Geometry check sheet. Reference: the model listing, model coordinates, mm. A direction names the side the tool comes from. Give positions to 0.01 mm unless a question says otherwise; leave off trailing zeros. Order: outer loops, then holes, each group sorted by start corner. A loop starts at its lowest first (then second) coordinate and runs counter-clockwise, first axis right, second up. Notation, with made-up numbers: M 32,-38.5 L 56,-38.5 A18 cw 56,-30.5 Z; hole C 54,8.5 d11. An arc over 180 degrees is marked long. Answer as a JSON object with one key per item and string values. Group by question number.
from build123d import *

# Parameters (mm, degrees)
SKETCH_W          = 3.32
SKETCH_H          = 32.28
PAD_DEPTH         = 3
PAD001_DEPTH      = 4
SKETCH002_W       = 3.32
SKETCH002_H       = 2
PAD002_DEPTH      = 2.01
FILLET_R          = 1.99
FILLET001_R       = 1.99
SKETCH003_W       = 11.8
SKETCH003_H       = 6.88
PAD003_DEPTH      = 1.5
SKETCH006_W       = 4.25
SKETCH006_H       = 4.4
PAD005_DEPTH      = 1.56
PAD005_DEPTH_BACK = 1.56
SKETCH007_W       = 2.24
SKETCH007_H       = 6.88
PAD006_DEPTH      = 0.92
POCKET_DEPTH      = 5
SKETCH009_R       = 0.72
PAD007_DEPTH      = 5
SKETCH010_R       = 0.72
PAD008_DEPTH      = 5
SKETCH011_R       = 0.8
POCKET001_DEPTH   = 5
SKETCH012_R       = 0.95
POCKET002_DEPTH   = 5


with BuildPart() as part:
    # Sketch → Pad (new body)
    with BuildSketch(Plane.XY):
        Rectangle(SKETCH_W, SKETCH_H)
    extrude(amount=PAD_DEPTH)

    # Sketch001 (on Face5 of Pad) → Pad001 (join)
    with BuildSketch(Plane(origin=(0, 0, 0), x_dir=(1, 0, 0), z_dir=(0, 0, -1))):
        Polygon((1.66, 6.275), (1.66, 11.275), (0, 11.275), (0, 9.385), (-1.66, 9.385), (-1.66, 7.965), (0, 7.965), (0, 6.275), align=None)
    pad001 = extrude(amount=PAD001_DEPTH)

    # Mirrored: Pad001 across Sketch001 H_Axis
    add(pad001.mirror(Plane(origin=(0, 0, 0), x_dir=(0, 0, -1), z_dir=(0, -1, 0))))

    # Sketch002 (on Face6 of Mirrored) → Pad002 (join)
    with BuildSketch(Plane.XZ.offset(16.14)):
        with Locations((0, 0.5)):
            Rectangle(SKETCH002_W, SKETCH002_H)
    pad002 = extrude(amount=PAD002_DEPTH)

    # Fillet
    fillet_edges = [part.edges().sort_by_distance(p)[0] for p in [
        (0, -18.15, 1.5),
    ]]
    fillet(fillet_edges, radius=FILLET_R)

    # Mirrored001: Pad002 across XZ
    add(pad002.mirror(Plane.XZ))

    # Fillet001
    fillet001_edges = [part.edges().sort_by_distance(p)[0] for p in [
        (0, 18.15, 1.5),
    ]]
    fillet(fillet001_edges, radius=FILLET001_R)

    # Sketch003 (on Face23 of Fillet001) → Pad003 (join)
    with BuildSketch(Plane(origin=(0, 0, -0.5), x_dir=(1, 0, 0), z_dir=(0, 0, -1))):
        with Locations((-1.64, 19.58)):
            Rectangle(SKETCH003_W, SKETCH003_H)
    pad003 = extrude(amount=PAD003_DEPTH)

    # Mirrored002: Pad003 across XZ
    add(pad003.mirror(Plane.XZ))

    # Sketch006 → Pad005 (join, two sides)
    with BuildSketch(Plane.XZ) as pad005_sk:
        with Locations((2.125, -0.7)):
            Rectangle(SKETCH006_W, SKETCH006_H)
    extrude(amount=PAD005_DEPTH)
    extrude(pad005_sk.sketch, amount=-PAD005_DEPTH_BACK)

    # Sketch007 (on Face56 of Pad005) → Pad006 (join)
    with BuildSketch(Plane(origin=(0, 0, -2), x_dir=(1, 0, 0), z_dir=(0, 0, -1))):
        with Locations((3.14, 19.58)):
            Rectangle(SKETCH007_W, SKETCH007_H)
    pad006 = extrude(amount=PAD006_DEPTH)

    # Mirrored003: Pad006 across XZ
    add(pad006.mirror(Plane.XZ))

    # Sketch008 (on Face43 of Mirrored003) → Pocket (cut)
    with BuildSketch(Plane.XY.offset(-0.5)):
        Polygon((4.26, -16.14), (4.26, -23.02), (-0.14, -23.02), align=None)
    pocket = extrude(amount=-POCKET_DEPTH, mode=Mode.SUBTRACT)

    # Mirrored004: Pocket across XZ
    add(pocket.mirror(Plane.XZ), mode=Mode.SUBTRACT)

    # Sketch009 (on Face59 of Mirrored004) → Pad007 (join)
    with BuildSketch(Plane(origin=(0, -16.14, 0), x_dir=(-1, 0, 0), z_dir=(0, 1, 0))):
        with Locations((-3.54, -2.2)):
            Circle(SKETCH009_R)
    pad007 = extrude(amount=PAD007_DEPTH)

    # Mirrored005: Pad007 across XZ
    add(pad007.mirror(Plane.XZ))

    # Sketch010 (on Face35 of Mirrored005) → Pad008 (join)
    with BuildSketch(Plane(origin=(0, 1.56, 0), x_dir=(-1, 0, 0), z_dir=(0, 1, 0))):
        with Locations((-3.53, -2.18)):
            Circle(SKETCH010_R)
    pad008 = extrude(amount=PAD008_DEPTH)

    # Mirrored006: Pad008 across XZ
    add(pad008.mirror(Plane.XZ))

    # Sketch011 (on Face2 of Mirrored006) → Pocket001 (cut)
    with BuildSketch(Plane.XY.offset(-0.5)):
        with Locations((-5.74, 20.12)):
            Circle(SKETCH011_R)
    pocket001 = extrude(amount=-POCKET001_DEPTH, mode=Mode.SUBTRACT)

    # Mirrored007: Pocket001 across XZ
    add(pocket001.mirror(Plane.XZ), mode=Mode.SUBTRACT)

    # Sketch012 (on Face2 of Mirrored007) → Pocket002 (cut)
    with BuildSketch(Plane.XY.offset(-0.5)):
        with Locations((-1.81, 20.12)):
            Circle(SKETCH012_R)
    pocket002 = extrude(amount=-POCKET002_DEPTH, mode=Mode.SUBTRACT)

    # Mirrored008: Pocket002 across XZ
    add(pocket002.mirror(Plane.XZ), mode=Mode.SUBTRACT)


solid = part.part
1. Release check for a two-part mould opening along Y. For faces 1 (the flat face through (2.03, -19.63, -1.42)), 2 (the flat face through (0, 0, -1)), 3 (the cylindrical face through (0.023, 17.552, 0.933)), 4 (the flat face through (0, 10, -2)) record: released by +Y, released by -Y, zero draft, split by the parting line, or undercut.
2. Thickness scan on line 1 along Y through (x, z) = (-5.74, -1.3); line 2 along Y through (x, z) = (-1.81, -1.35); line 3 along X through (y, z) = (-11, 1.5). Record the ranges inside material, lowest first. Write a range as [from, to].
3. Cross-section at D-D (y = -20.12). Record the cut outline in (x, z), and give its area (3 significant figures).
4. Cross-section at C-C (x = -2.25). Record the cut outline in (y, z), and give its area (3 significant figures).
5. Cross-section at B-B (y = -13). Record the cut outline in (x, z).
6. Access from +Z, -Z, +X, -X, +Y, -Y to the whole of each face (thin tool, end or side, straight path). Record for faces 5 (the cylindrical face through (2.843, -4.025, -1.964)), 6 (the flat face through (2.03, 19.63, -1.42)), 7 (the flat face through (4, 6.56, -2)), 8 (the flat face through (0, -16.14, 2)), 9 (the flat face through (-1, -7.965, -2)).
7. Cross-section at A-A (x = -4.5). Record the cut outline in (y, z), and give its area (3 significant figures).
8. Depth check by flat-ended pin: pin 1 (0.8 mm diameter, centred on x = 4, z = -2.5, fed in from -Y); pin 2 (3.5 mm diameter, centred on x = 2.5, y = -0.5, fed in from -Z); pin 3 (5 mm diameter, centred on x = -2.5, y = 12, fed in from +Z); pin 4 (2 mm diameter, centred on x = 3, z = -1.5, fed in from -Y). Enter the tip coordinate at first touch or a pass-through.
Report:
{
 "1": {"face 1": "released by -Y", "face 2": "undercut", "face 3": "released by +Y", "face 4": "undercut"},
 "2": {"line 1": "y = [-23.02, -20.92], [-19.32, -16.14], [16.14, 19.32], [20.92, 23.02]", "line 2": "y = [-23.02, -21.07], [-19.17, -16.14], [16.14, 19.17], [21.07, 23.02]", "line 3": "x = [-1.66, 1.66]"},
 "3": {"outline": "M -7.54,-2 L -6.54,-2 L -6.54,-0.5 L -7.54,-0.5 Z; M -4.94,-2 L -2.76,-2 L -2.76,-0.5 L -4.94,-0.5 Z; M -0.86,-2 L 1.71,-2 L 1.71,-0.5 L -0.86,-0.5 Z", "area": "8.63 mm2"},
 "4": {"outline": "M -23.02,-2 L -20.96,-2 L -20.96,-0.5 L -23.02,-0.5 Z; M -19.28,-2 L -16.14,-2 L -16.14,-0.5 L -19.28,-0.5 Z; M 16.14,-2 L 19.28,-2 L 19.28,-0.5 L 16.14,-0.5 Z; M 20.96,-2 L 23.02,-2 L 23.02,-0.5 L 20.96,-0.5 Z", "area": "15.6 mm2"},
 "5": {"outline": "M -1.66,0 L 1.66,0 L 1.66,3 L -1.66,3 Z; C 3.54,-2.2 d1.44"},
 "6": {"face 5": "none", "face 6": "+Z, -Z, +X, +Y", "face 7": "+Z, -Z, +X", "face 8": "+Z, +X, -X, -Y", "face 9": "-Z, -X"},
 "7": {"outline": "M -23.02,-2 L -16.14,-2 L -16.14,-0.5 L -23.02,-0.5 Z; M 16.14,-2 L 23.02,-2 L 23.02,-0.5 L 16.14,-0.5 Z", "area": "20.6 mm2"},
 "8": {"pin 1": "stops at y = -17.17", "pin 2": "stops at z = -2.9", "pin 3": "stops at z = 3", "pin 4": "stops at y = -19.67"}
}
